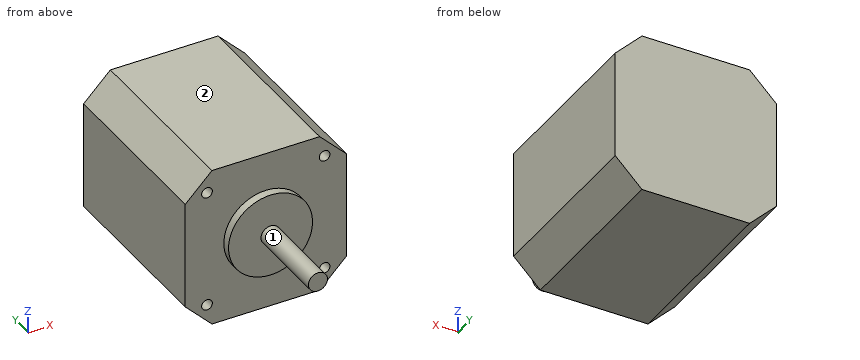
```python
from build123d import *

# Parameters (mm, degrees)
F0_W     = 42.2
F0_H     = 42.2
F1_DEPTH = 23.6
F2_SIZE  = 7
F3_R     = 2.5
F4_DEPTH = 24.2
F5_R     = 11
F6_DEPTH = 2.2
F7_R     = 1.4
F8_DEPTH = 10


with BuildPart() as f1:
    # F0 (on Front) → F1 (new body, symmetric)
    with BuildSketch(Plane.XZ):
        Rectangle(F0_W, F0_H)
    extrude(amount=F1_DEPTH, both=True)

    # F2
    f2_edges = [f1.edges().sort_by_distance(p)[0] for p in [
        (21.1, 0, 21.1),
        (-21.1, 0, 21.1),
        (21.1, 0, -21.1),
        (-21.1, 0, -21.1),
    ]]
    chamfer(f2_edges, length=F2_SIZE)

    # F3 (on face) → F4 (join)
    with BuildSketch(Plane.XZ.offset(23.6)):
        Circle(F3_R)
    extrude(amount=F4_DEPTH)

    # F5 (on face) → F6 (join)
    with BuildSketch(Plane.XZ.offset(23.6)):
        Circle(F5_R)
    extrude(amount=F6_DEPTH)

    # F7 (on face) → F8 (cut)
    with BuildSketch(Plane.XZ.offset(23.6)):
        with Locations((-15.4, -15.4)):
            Circle(F7_R)
        with Locations((-15.4, 15.4)):
            Circle(F7_R)
        with Locations((15.4, -15.4)):
            Circle(F7_R)
        with Locations((15.4, 15.4)):
            Circle(F7_R)
    extrude(amount=-F8_DEPTH, mode=Mode.SUBTRACT)


solid = f1.part
```
Input: part model. Units: mm. Frame: model coordinates. Face numbers are marked on the shaded views. A direction names the side the tool comes from. Coordinates: 2 decimals unless noted, no trailing zeros. Write each loop counter-clockwise with the first axis right and the second up, starting at its lowest first coordinate (ties: lowest second). Pieces come first, ordered by that corner, then holes.
1) Pin query (flat end, axial travel): pin 1 Ø2 at (x, z) = (-15.5, -16) entering from -Y; pin 2 Ø24 at (x, z) = (2.5, -4) entering from -Y; pin 3 Ø2.5 at (x, z) = (-15.4, 15.4) entering from -Y; pin 4 Ø3 at (x, z) = (-2.5, -10.5) entering from -Y. Return the tip coordinate at first contact, or that it passes through.
2) Set-up query: the marked faces 1 and 2. Return all of +Z, -Z, +X, -X, +Y, -Y with unobstructed straight access to the full face (end or side cutting, diameter ignored); none if empty.
3) Material intervals for line 1 along Z through (x, y) = (15, -21); line 2 along Z through (x, y) = (-15.4, -16.5); line 3 along Y through (x, z) = (2, 15.5), sorted ascending.
4) Section D-D on y = -11. Output: boundary loops of the cut face in (x, z).
5) Section B-B on x = -15.4. Output: boundary loops of the cut face in (y, z), and give its area (3 significant figures).
6) Section C-C on z = -15.4. Output: boundary loops of the cut face in (x, y).
7) Section A-A on y = -19. Output: boundary loops of the cut face in (x, z), and give its area (3 significant figures).
Check result:
1. pin 1: stops at y = -23.6
1. pin 2: stops at y = -47.8
1. pin 3: stops at y = -13.6
1. pin 4: stops at y = -25.8
2. face 1: -Y
2. face 2: +Z, +X, -X, +Y, -Y
3. line 1: z = -20.2 to -16.74, -14.06 to 14.06, 16.74 to 20.2
3. line 2: z = -19.8 to -16.8, -14 to 14, 16.8 to 19.8
3. line 3: y = -23.6 to 23.6
4. outline: (-21.1, -14.1) - (-14.1, -21.1) - (14.1, -21.1) - (21.1, -14.1) - (21.1, 14.1) - (14.1, 21.1) - (-14.1, 21.1) - (-21.1, 14.1) - close
5. outline: (-23.6, -19.8) - (23.6, -19.8) - (23.6, 19.8) - (-23.6, 19.8) - (-23.6, 16.8) - (-13.6, 16.8) - (-13.6, 14) - (-23.6, 14) - (-23.6, -14) - (-13.6, -14) - (-13.6, -16.8) - (-23.6, -16.8) - close
5. area: 1,810 mm2
6. outline: (-19.8, -23.6) - (-16.8, -23.6) - (-16.8, -13.6) - (-14, -13.6) - (-14, -23.6) - (14, -23.6) - (14, -13.6) - (16.8, -13.6) - (16.8, -23.6) - (19.8, -23.6) - (19.8, 23.6) - (-19.8, 23.6) - close
7. outline: (-21.1, -14.1) - (-14.1, -21.1) - (14.1, -21.1) - (21.1, -14.1) - (21.1, 14.1) - (14.1, 21.1) - (-14.1, 21.1) - (-21.1, 14.1) - close; hole circle Ø2.8 at (-15.4, -15.4); hole circle Ø2.8 at (-15.4, 15.4); hole circle Ø2.8 at (15.4, -15.4); hole circle Ø2.8 at (15.4, 15.4)
7. area: 1,660 mm2
